For this review, take the finished solid that the model builds, in its own axes (mm). A direction names the side the tool comes from. Round coordinates to 2 decimals unless told otherwise and drop trailing zeros. Write each loop counter-clockwise with the first axis right and the second up, starting at its lowest first coordinate (ties: lowest second). Pieces come first, ordered by that corner, then holes. Notation, with made-up numbers: (0.5, 20.5) -> (42.5, 20.5) arc R16 ccw to (42.5, 50.5) -> close; hole circle Ø2 at (19, 6.25). An arc over 180 degrees is marked (long way). Answer in a Markdown table with one row per item.
from build123d import *

# Parameters (mm, degrees)
SKETCH_1_W                         = 48.1
SKETCH_1_H                         = 50
SM_BASE_FLANGE_1_DEPTH             = 1.2
SM_EDGE_FLANGE_1_STRIP_W           = 6.2732
SM_EDGE_FLANGE_1_STRIP_H           = 1.2
SM_EDGE_FLANGE_1_STRIP_CUT_DEPTH   = 50
SM_EDGE_FLANGE_1_STRIP_2_W         = 6.2732
SM_EDGE_FLANGE_1_STRIP_2_H         = 1.2
SM_EDGE_FLANGE_1_STRIP_CUT_2_DEPTH = 50
SM_EDGE_FLANGE_1_DEPTH             = 50
SM_EDGE_FLANGE_1_BEND_DEPTH        = 50
CUT_EXTRUDE_1_DEPTH                = 10
SKETCH_17_R                        = 1
CUT_EXTRUDE_2_DEPTH                = 59.631817301
FILLET_1_R                         = 2


# Sheet-metal steps are written as plain solids
with BuildPart() as part:
    # Sketch 1 → 基材-凸緣1 (new body)
    with BuildSketch(Plane.XY):
        Rectangle(SKETCH_1_W, SKETCH_1_H)
    extrude(amount=-SM_BASE_FLANGE_1_DEPTH)

    # 邊線-凸緣1 strip (across the edge) → 邊線-凸緣1 strip cut (cut)
    with BuildSketch(Plane(origin=(24.05, 25, -1.2), x_dir=(-1, 0, 0), z_dir=(0, -1, 0))):
        with Locations((-2.4, -0.6)):
            Rectangle(SM_EDGE_FLANGE_1_STRIP_W, SM_EDGE_FLANGE_1_STRIP_H)
    extrude(amount=SM_EDGE_FLANGE_1_STRIP_CUT_DEPTH, mode=Mode.SUBTRACT)

    # 邊線-凸緣1 strip 2 (across the edge) → 邊線-凸緣1 strip cut 2 (cut)
    with BuildSketch(Plane(origin=(-24.05, -25, -1.2), x_dir=(1, 0, 0), z_dir=(0, 1, 0))):
        with Locations((-2.4, -0.6)):
            Rectangle(SM_EDGE_FLANGE_1_STRIP_2_W, SM_EDGE_FLANGE_1_STRIP_2_H)
    extrude(amount=SM_EDGE_FLANGE_1_STRIP_CUT_2_DEPTH, mode=Mode.SUBTRACT)

    # 邊線-凸緣1 section (across the edge) → 邊線-凸緣1 (add)
    with BuildSketch(Plane(origin=(24.05, 25, -1.2), x_dir=(-1, 0, 0), z_dir=(0, -1, 0))):
        with BuildLine():
            Line((-1.2, 0.7366), (-1.2, 15))
            Line((-1.2, 15), (0, 15))
            Line((0, 15), (0, 0.7366))
            ThreePointArc((0, 0.7366), (0.215745145, 0.215745145), (0.7366, 0))
            Line((0.7366, 0), (0.7366, -1.2))
            ThreePointArc((0.7366, -1.2), (-0.632782992, -0.632782992), (-1.2, 0.7366))
        make_face()
    extrude(amount=SM_EDGE_FLANGE_1_DEPTH)

    # 邊線-凸緣1 section 2 (across the edge) → 邊線-凸緣1 bend (add)
    with BuildSketch(Plane(origin=(-24.05, -25, -1.2), x_dir=(1, 0, 0), z_dir=(0, 1, 0))):
        with BuildLine():
            Line((-1.2, 0.7366), (-1.2, 15))
            Line((-1.2, 15), (0, 15))
            Line((0, 15), (0, 0.7366))
            ThreePointArc((0, 0.7366), (0.215745145, 0.215745145), (0.7366, 0))
            Line((0.7366, 0), (0.7366, -1.2))
            ThreePointArc((0.7366, -1.2), (-0.632782992, -0.632782992), (-1.2, 0.7366))
        make_face()
    extrude(amount=SM_EDGE_FLANGE_1_BEND_DEPTH)

    # 草圖14 → 除料-伸長1 (cut)
    with BuildSketch(Plane.XY):
        with BuildLine():
            Line((-7.752874967, 18), (7.752874967, 18))
            ThreePointArc((7.752874967, 18), (9.581283984, 16.810506303), (9.234812, 14.656920467))
            Line((9.234812, 14.656920467), (1.481937033, 6.10249592))
            ThreePointArc((1.481937033, 6.10249592), (0, 5.445575453), (-1.481937033, 6.10249592))
            Line((-1.481937033, 6.10249592), (-9.234812, 14.656920467))
            ThreePointArc((-9.234812, 14.656920467), (-9.581283984, 16.810506303), (-7.752874967, 18))
        make_face()
        with BuildLine():
            Line((-16.3134, 8.347649749), (-16.3134, -8.347649749))
            ThreePointArc((-16.3134, -8.347649749), (-15.033165911, -10.213644666), (-12.831462967, -9.690729281))
            Line((-12.831462967, -9.690729281), (-5.265988, -1.343079533))
            ThreePointArc((-5.265988, -1.343079533), (-4.747925033, 0), (-5.265988, 1.343079533))
            Line((-5.265988, 1.343079533), (-12.831462967, 9.690729281))
            ThreePointArc((-12.831462967, 9.690729281), (-15.033165911, 10.213644666), (-16.3134, 8.347649749))
        make_face()
        with BuildLine():
            Line((-7.752874967, -18), (7.752874967, -18))
            ThreePointArc((7.752874967, -18), (9.581283984, -16.810506303), (9.234812, -14.656920467))
            Line((9.234812, -14.656920467), (1.481937033, -6.10249592))
            ThreePointArc((1.481937033, -6.10249592), (0, -5.445575453), (-1.481937033, -6.10249592))
            Line((-1.481937033, -6.10249592), (-9.234812, -14.656920467))
            ThreePointArc((-9.234812, -14.656920467), (-9.581283984, -16.810506303), (-7.752874967, -18))
        make_face()
        with BuildLine():
            Line((16.3134, 8.347649749), (16.3134, -8.347649749))
            ThreePointArc((16.3134, -8.347649749), (15.033165911, -10.213644666), (12.831462967, -9.690729281))
            Line((12.831462967, -9.690729281), (5.265988, -1.343079533))
            ThreePointArc((5.265988, -1.343079533), (4.747925033, 0), (5.265988, 1.343079533))
            Line((5.265988, 1.343079533), (12.831462967, 9.690729281))
            ThreePointArc((12.831462967, 9.690729281), (15.033165911, 10.213644666), (16.3134, 8.347649749))
        make_face()
    extrude(amount=-CUT_EXTRUDE_1_DEPTH, mode=Mode.SUBTRACT)

    # 草圖17 → 除料-伸長2 (cut, through all)
    with BuildSketch(Plane(origin=(25.25, 0, 0), x_dir=(0, 0, -1), z_dir=(1, 0, 0))):
        with Locations((5, 20)):
            Circle(SKETCH_17_R)
        with Locations((5.000020411, -15)):
            Circle(SKETCH_17_R)
        with Locations((12, 2.5)):
            Circle(SKETCH_17_R)
    extrude(amount=-CUT_EXTRUDE_2_DEPTH, mode=Mode.SUBTRACT)

    # 圓角1
    fillet_1_edges = [part.edges().sort_by_distance(p)[0] for p in [
        (24.65, 25, -16.2),
        (24.65, -25, -16.2),
        (-24.65, -25, -16.2),
        (-24.65, 25, -16.2),
    ]]
    fillet(fillet_1_edges, radius=FILLET_1_R)


solid = part.part
1) For line 1 (Y direction, x = -24.45, z = -5); line 2 (X direction, y = 1.5, z = -8.75); line 3 (Z direction, x = -21, y = -10.5), list the stretches that pass through material, from the lowest coordinate up. Write a range as [from, to].
Solved:
| item | result |
|---|---|
| line 1 | [-25, -16], [-14, 19], [21, 25] |
| line 2 | [-25.25, -24.05], [24.05, 25.25] |
| line 3 | [-1.2, 0] |
2) Consider section B-B on y = 20. State the section outline as (x, z) points, then the cut area to 3 significant figures.
Solved:
| item | result |
|---|---|
| outline | (-25.25, -16.2) -> (-24.05, -16.2) -> (-24.05, -6) -> (-25.25, -6) -> close; (-25.25, -4) -> (-24.05, -4) -> (-24.05, -1.94) arc R0.74 cw to (-23.31, -1.2) -> (23.31, -1.2) arc R0.74 cw to (24.05, -1.94) -> (24.05, -4) -> (25.25, -4) -> (25.25, -1.94) arc R1.94 ccw to (23.31, 0) -> (-23.31, 0) arc R1.94 ccw to (-25.25, -1.94) -> close; (24.05, -16.2) -> (25.25, -16.2) -> (25.25, -6) -> (24.05, -6) -> close |
| area | 90.4 mm² |
3) For faces 1 (the cylindrical face through (-24.64, 24.43, -15.6)), 2 (the flat face through (-5.304, -10.32, -0.592)), 3 (the flat face through (24.05, 0, -9)), list the 3-axis set-ups (+Z, -Z, +X, -X, +Y, -Y) from which the entire face can be reached by the end or side of a thin tool; tool diameter is ignored.
Solved:
| item | result |
|---|---|
| face 1 | -Z, +X, -X, +Y |
| face 2 | +Z, -Z |
| face 3 | -Z, +Y, -Y |
4) Consider section C-C on z = -5. State the section outline as (x, y) points.
Solved:
| item | result |
|---|---|
| outline | (-25.25, -25) -> (-24.05, -25) -> (-24.05, -16) -> (-25.25, -16) -> close; (-25.25, -14) -> (-24.05, -14) -> (-24.05, 19) -> (-25.25, 19) -> close; (-25.25, 21) -> (-24.05, 21) -> (-24.05, 25) -> (-25.25, 25) -> close; (24.05, -25) -> (25.25, -25) -> (25.25, -16) -> (24.05, -16) -> close; (24.05, -14) -> (25.25, -14) -> (25.25, 19) -> (24.05, 19) -> close; (24.05, 21) -> (25.25, 21) -> (25.25, 25) -> (24.05, 25) -> close |
5) Clearance check with flat-ended pins moving along their axes: pin 1 Ø1.5 at (x, y) = (-19.5, 5.5) entering from +Z; pin 2 Ø1 at (x, y) = (10, -17) entering from -Z; pin 3 Ø1.2 at (y, z) = (-15, -5) entering from +X; pin 4 Ø1 at (y, z) = (3, -0.5) entering from +X. State where each tip first meets the part, or that it passes through.
Solved:
| item | result |
|---|---|
| pin 1 | z = 0 |
| pin 2 | z = -1.2 |
| pin 3 | through |
| pin 4 | x = 25.01 |
6) Mouldability with a two-part tool opening along X and no side actions: class faces 4 (the flat face through (0, 18, -1)), 5 (the cylindrical face through (24.64, -24.43, -15.6)), 6 (the flat face through (-25.25, 0, -9)) as pulls with the +X half, pulls with the -X half, needs draft (parallel to the pull), parting line crosses it, or undercut.
Solved:
| item | result |
|---|---|
| face 4 | undercut |
| face 5 | needs draft |
| face 6 | pulls with the -X half |
7) Consider section A-A on z = -10. State the section outline as (x, y) points.
Solved:
| item | result |
|---|---|
| outline | (-25.25, -25) -> (-24.05, -25) -> (-24.05, 25) -> (-25.25, 25) -> close; (24.05, -25) -> (25.25, -25) -> (25.25, 25) -> (24.05, 25) -> close |
8) Consider section D-D on x = -11. State the section outline as (y, z) points.
Solved:
| item | result |
|---|---|
| outline | (-25, -1.2) -> (-7.67, -1.2) -> (-7.67, 0) -> (-25, 0) -> close; (7.67, -1.2) -> (25, -1.2) -> (25, 0) -> (7.67, 0) -> close |
